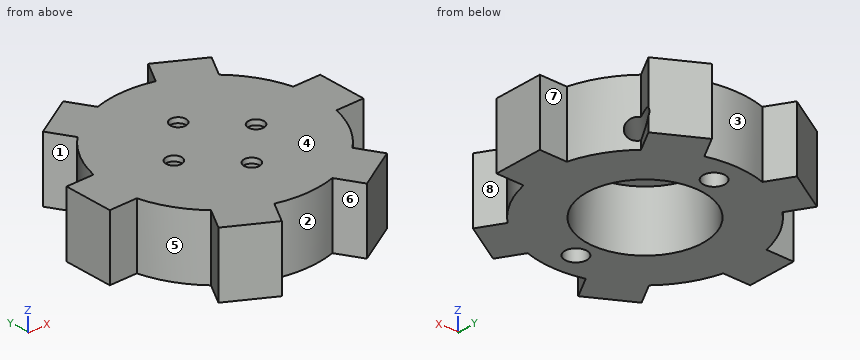
Autodesk Inventor part; units mm, degrees
ref_plane "РабПлоскость1" through (-24.7024, -23.7395, 10.5) normal (0, 0, 1) x (1, 0, 0)
ref_plane "РабПлоскость2" through (-24.7024, -23.7395, 9) normal (0, 0, -1) x (0, 1, 0)
ref_plane "YZ Plane" through (0, 0, 0) normal (1, 0, 0) x (0, 1, 0)
sketch "Эскиз1" plane through (0, 0, 0) normal (0, 0, 1) x (1, 0, 0)
  line L0 (0, 0) -> (34.5691, 5.4752) construction
  line L1 (0, 0) -> (35, 0) construction
  line L2 (0, 0) -> (34.5691, -5.4752) construction
  circle A0 centre (0, 0) radius 11.25
  circle A1 centre (0, 0) radius 15
  circle A2 centre (0, 0) radius 20
  circle A3 centre (0, 0) radius 30.0525
  circle A4 centre (0, 0) radius 32.0038
  circle A5 centre (0, 0) radius 35
  line L3 (0, 0) -> (17.5, -30.3109) construction
  circle A6 centre (0, -8) radius 1.5
  circle A7 centre (-8, 0) radius 1.5
  line L4 (0, 0) -> (-35, 0) construction
  line L5 (-29.6307, -4.693) -> (-19.4416, -4.693) construction
  line L6 (-29.6307, -4.693) -> (-19.4416, -4.693)
  line L7 (-29.6839, -4.693) -> (-29.6839, 4.693)
  line L8 (-19.4416, 4.693) -> (-34.6839, 4.693) construction
  line L9 (-19.4416, -4.693) -> (-34.6839, -4.693) construction
  line L10 (10.751, 28.0074) -> (5.6565, 19.1834) construction
  line L11 (5.6565, 19.1834) -> (13.2777, 32.3837) construction
  line L12 (-5.6565, 19.1834) -> (-13.2777, 32.3837) construction
  circle A8 centre (0, 8) radius 1.5
  line L13 (0, 0) -> (-17.5, 30.3109) construction
  line L14 (-5.6565, 19.1834) -> (-13.2777, 32.3837)
  line L15 (0, 0) -> (17.5, 30.3109) construction
  line L16 (0, 0) -> (-17.5, -30.3109) construction
  line L17 (5.6565, 19.1834) -> (13.2777, 32.3837)
  line L18 (13.3758, 26.5536) -> (16.0133, 31.1219)
  line L19 (16.3082, 24.8605) -> (18.9457, 29.4289)
  line L20 (18.9457, 29.4289) -> (17.4457, 26.8308) construction
  line L21 (29.6307, 4.693) -> (19.4416, 4.693)
  line L22 (18.8796, -23.3144) -> (13.7851, -14.4904) construction
  line L23 (13.7851, -14.4904) -> (21.4063, -27.6907) construction
  line L24 (29.6839, 4.693) -> (29.6839, 1.693)
  line L25 (29.6839, 4.693) -> (29.6839, -4.693)
  line L26 (29.6839, -4.693) -> (29.6839, -1.693) construction
  circle A9 centre (8, 0) radius 1.5
  line L27 (-18.8796, 23.3144) -> (-13.7851, 14.4904) construction
  line L28 (-13.7851, 14.4904) -> (-21.4063, 27.6907) construction
  line L29 (-18.8796, 23.3144) -> (-13.7851, 14.4904)
  line L30 (-13.7851, 14.4904) -> (-21.4063, 27.6907)
  line L31 (-18.9063, 23.3605) -> (-10.7777, 28.0536)
  line L32 (-16.3082, 24.8605) -> (-18.9457, 29.4289)
  line L33 (-13.3758, 26.5536) -> (-16.0133, 31.1219)
  line L34 (-13.7851, -14.4904) -> (-21.4063, -27.6907) construction
  line L35 (-10.751, -28.0074) -> (-5.6565, -19.1834) construction
  line L36 (-13.7851, -14.4904) -> (-21.4063, -27.6907)
  line L37 (-10.751, -28.0074) -> (-5.6565, -19.1834)
  line L38 (13.7851, 14.4904) -> (21.4063, 27.6907) construction
  line L39 (21.4063, 27.6907) -> (20.1674, 25.5449) construction
  line L40 (10.7777, 28.0536) -> (18.9063, 23.3605)
  line L41 (13.7851, 14.4904) -> (21.4063, 27.6907)
  line L42 (10.751, 28.0074) -> (5.6565, 19.1834)
  line L43 (0, 0) -> (21.2118, 27.8399) construction
  line L44 (0, 0) -> (8, 0) construction
  line L45 (0, 0) -> (0, 8) construction
  line L46 (-10.7777, -28.0536) -> (-18.9063, -23.3605)
  line L47 (-13.3758, -26.5536) -> (-16.0133, -31.1219)
  line L48 (-16.3082, -24.8605) -> (-18.9457, -29.4289)
  line L49 (-5.6565, -19.1834) -> (-13.2777, -32.3837) construction
  line L50 (5.6565, -19.1834) -> (13.2777, -32.3837) construction
  line L51 (-5.6565, -19.1834) -> (-13.2777, -32.3837)
  line L52 (18.8796, -23.3144) -> (13.7851, -14.4904)
  line L53 (5.6565, -19.1834) -> (13.2777, -32.3837)
  line L54 (16.3082, -24.8605) -> (18.9457, -29.4289)
  line L55 (13.7851, -14.4904) -> (21.4063, -27.6907)
  line L56 (13.3758, -26.5536) -> (16.0133, -31.1219)
  line L57 (18.9063, -23.3605) -> (10.7777, -28.0536)
  line L58 (27.6414, 16.1308) -> (28.831, 19.8437)
  line L59 (24.938, 20.0584) -> (28.831, 19.8437)
  line L60 (24.7499, 20.2901) -> (25.3388, 24.1443)
  line L61 (21.4607, 23.742) -> (25.3388, 24.1443)
  line L62 (17.4457, 26.8308) -> (21.2118, 27.8399)
  line L63 (21.2384, 23.9411) -> (21.2118, 27.8399)
  line L64 (-19.4416, 4.693) -> (-34.6839, 4.693)
  line L65 (-17.4453, 26.8311) -> (-21.2113, 27.8403)
  line L66 (-21.238, 23.9415) -> (-21.2113, 27.8403)
  line L67 (-21.4603, 23.7424) -> (-25.3384, 24.1447)
  line L68 (-24.7496, 20.2905) -> (-25.3384, 24.1447)
  line L69 (-24.9377, 20.0588) -> (-28.8307, 19.8442)
  line L70 (-27.6411, 16.1312) -> (-28.8307, 19.8442)
  line L71 (-27.7903, 15.8727) -> (-31.6007, 15.0465)
  line L72 (-29.8401, 11.5678) -> (-31.6007, 15.0465)
  line L73 (-29.9467, 11.289) -> (-33.5789, 9.8719)
  line L74 (-31.2916, 6.7145) -> (-33.5789, 9.8719)
  line L75 (-31.3528, 6.4224) -> (-34.716, 4.45)
  line L76 (-29.6839, -1.693) -> (-34.959, -1.693)
  line L77 (-19.4416, -4.693) -> (-34.6839, -4.693)
  line L78 (-29.6839, 1.693) -> (-34.959, 1.693)
  line L79 (-31.959, 1.693) -> (-34.716, 4.45)
  line L80 (-31.9591, -1.6925) -> (-34.716, -4.4494)
  line L81 (-31.3529, -6.4219) -> (-34.716, -4.4494)
  line L82 (-31.2917, -6.714) -> (-33.5791, -9.8714)
  line L83 (-29.9469, -11.2885) -> (-33.5791, -9.8714)
  line L84 (-29.8403, -11.5673) -> (-31.6009, -15.046)
  line L85 (-27.7906, -15.8723) -> (-31.6009, -15.046)
  line L86 (-24.938, -20.0584) -> (-28.831, -19.8437)
  line L87 (-27.6414, -16.1308) -> (-28.831, -19.8437)
  line L88 (-17.4457, -26.8308) -> (-21.2118, -27.8399)
  line L89 (-21.2384, -23.9411) -> (-21.2118, -27.8399)
  line L90 (-21.4607, -23.742) -> (-25.3388, -24.1443)
  line L91 (-24.7499, -20.2901) -> (-25.3388, -24.1443)
  line L92 (-14.5138, -28.5236) -> (-13.5047, -32.2897)
  line L93 (-10.1149, -30.3634) -> (-13.5047, -32.2897)
  line L94 (-9.8313, -30.4564) -> (-8.2407, -34.016)
  line L95 (-5.1973, -31.579) -> (-8.2407, -34.016)
  line L96 (-4.9026, -31.6261) -> (-2.7702, -34.8902)
  line L97 (-0.1495, -32.0035) -> (-2.7702, -34.8902)
  line L98 (0.149, -32.0035) -> (2.7697, -34.8902)
  line L99 (-14.5133, 28.5238) -> (-13.5042, 32.2899)
  line L100 (-10.1144, 30.3635) -> (-13.5042, 32.2899)
  line L101 (-9.8308, 30.4565) -> (-8.2401, 34.0162)
  line L102 (-5.1968, 31.5791) -> (-8.2401, 34.0162)
  line L103 (14.5138, 28.5236) -> (13.5047, 32.2897)
  line L104 (10.1149, 30.3634) -> (13.5047, 32.2897)
  line L105 (9.8313, 30.4564) -> (8.2407, 34.016)
  line L106 (5.1973, 31.579) -> (8.2407, 34.016)
  line L107 (4.9026, 31.6261) -> (2.7702, 34.8902)
  line L108 (0.1495, 32.0035) -> (2.7702, 34.8902)
  line L109 (-4.9021, 31.6262) -> (-2.7697, 34.8902)
  line L110 (-0.149, 32.0035) -> (-2.7697, 34.8902)
  line L111 (14.5133, -28.5238) -> (13.5042, -32.2899)
  line L112 (5.1968, -31.5791) -> (8.2401, -34.0162)
  line L113 (9.8308, -30.4565) -> (8.2401, -34.0162)
  line L114 (10.1144, -30.3635) -> (13.5042, -32.2899)
  line L115 (17.4453, -26.8311) -> (21.2113, -27.8403)
  line L116 (21.238, -23.9415) -> (21.2113, -27.8403)
  line L117 (4.9021, -31.6262) -> (2.7697, -34.8902)
  line L118 (19.4416, -4.693) -> (34.6839, -4.693)
  line L119 (29.6839, -1.693) -> (34.959, -1.693)
  line L120 (21.4603, -23.7424) -> (25.3384, -24.1447)
  line L121 (24.7496, -20.2905) -> (25.3384, -24.1447)
  line L122 (24.9377, -20.0588) -> (28.8307, -19.8442)
  line L123 (27.6411, -16.1312) -> (28.8307, -19.8442)
  line L124 (27.7903, -15.8727) -> (31.6007, -15.0465)
  line L125 (29.9467, -11.289) -> (33.5789, -9.8719)
  line L126 (31.2916, -6.7145) -> (33.5789, -9.8719)
  line L127 (31.3528, -6.4224) -> (34.716, -4.45)
  line L128 (31.959, -1.693) -> (34.716, -4.45)
  line L129 (29.8401, -11.5678) -> (31.6007, -15.0465)
  line L130 (34.5691, 5.4752) -> (29.6307, 4.693) construction
  line L131 (19.4416, 4.693) -> (34.6839, 4.693)
  line L132 (34.6839, 4.693) -> (29.6839, 4.693) construction
  line L133 (29.6839, 1.693) -> (34.959, 1.693)
  line L134 (29.8403, 11.5673) -> (31.6009, 15.046)
  line L135 (31.2917, 6.714) -> (33.5791, 9.8714)
  line L136 (31.9591, 1.6925) -> (34.716, 4.4494)
  line L137 (31.3529, 6.4219) -> (34.716, 4.4494)
  line L138 (29.9469, 11.2885) -> (33.5791, 9.8714)
  line L139 (27.7906, 15.8723) -> (31.6009, 15.046)
  circle A10 centre (0, 0) radius 36.5
  line L140 (0, 0) -> (-24.7487, 24.7487) construction
  line L141 (0, 0) -> (35, 0) construction
  line L142 (0, 0) -> (-24.6962, 0) construction
  line L143 (-24.6962, -4.693) -> (-24.6962, 4.693)
  line L144 (-8.2838, -23.734) -> (-16.4124, -19.041)
  line L145 (16.4124, -19.041) -> (8.2838, -23.734)
  line L146 (24.6962, 4.693) -> (24.6962, -4.693)
  line L147 (8.2838, 23.734) -> (16.4124, 19.041)
  line L148 (-16.4124, 19.041) -> (-8.2838, 23.734)
  line L149 (0, 0) -> (21.2503, 21.2503) construction
  line L150 (0, 0) -> (30.0525, 0) construction
  line L151 (14.1421, 14.1421) -> (23.5912, 4.693)
  line L152 (23.5912, 4.693) -> (-6.168, 34.4522)
  circle A11 centre (0, 15) radius 2.1
  circle A12 centre (0, -15) radius 2.1
  point P0 (0, 0)
  point P1 (18.9062, 23.3604)
  point P2 (18.9055, 23.3609)
  point P3 (10.7784, 28.0531)
  point P4 (-10.7784, 28.0531)
  point P5 (-18.9055, 23.3609)
  point P6 (-18.9062, 23.3604)
  point P7 (-29.6838, 4.693)
  point P8 (-29.6839, 4.6922)
  point P9 (-29.6839, -4.6922)
  point P10 (-18.9055, -23.3609)
  point P11 (-10.7784, -28.0531)
  point P12 (-10.7776, -28.0534)
  point P13 (10.7776, -28.0534)
  point P14 (10.7784, -28.0531)
  point P15 (18.9055, -23.3609)
  point P16 (29.6839, -4.6922)
  point P17 (29.6839, 4.6922)
  point P18 (29.6838, 4.693)
  point P19 (-29.6838, -4.693)
  point P20 (-18.9062, -23.3604)
  point P21 (18.9062, -23.3604)
  point P22 (29.6838, -4.693)
  point P23 (10.7776, 28.0534)
  point P24 (-10.7776, 28.0534)
  point P25 (-24.6962, 4.693)
  point P26 (24.6962, -4.693)
  dimension "d10" = 70
  dimension "d21" = 60.105
  dimension "d31" = 30
  dimension "d11" = 40
  dimension "d12" = 9
  dimension "d13" = 5
  dimension "d14" = 360
  dimension "d15" = 360
  dimension "d16" = 5
  dimension "d17" = 90
  dimension "d18" = 3
  dimension "d19" = 3
  dimension "d20" = 360
  dimension "d22" = 3
  dimension "d23" = 45
  dimension "d24" = 45.392
  dimension "d25" = 360
  dimension "d26" = 22.5
  dimension "d27" = 8
  dimension "d28" = 3
  dimension "d29" = 8
  dimension "d30" = 3
  dimension "d32" = 73
  dimension "d45" = 135
  dimension "d48" = 360
  dimension "d54" = 45
  dimension "d63" = 4.2
extrude "Выдавливание1" add sketch "Эскиз1" along normal blind 11.5 contours A1 A12 A11 | A11 A1 | A1 A11 | A12 A1 | A1 A12 | A2
extrude "Выдавливание4" add sketch "Эскиз1" along normal blind 1 from surface at 11.5 contours A0 | A1 A12 A11 | A11 A1 | A1 A11 | A12 A1 | A1 A12 | A2
ref_plane "РабПлоскость1" through (-24.7024, -23.7395, 10.5) normal (0, 0, 1) x (1, 0, 0)
ref_plane "РабПлоскость2" through (-24.7024, -23.7395, 9) normal (0, 0, -1) x (0, 1, 0)
extrude "Выдавливание7" add sketch "Эскиз1" along normal blind 12.5 contours A2 L21 L146 L118 | L52 L145 L53 A2 | A2 L17 L152 L41 | L152 L17 L147 L41 | L37 L144 L36 A2 | A2 L29 L148 L14 | L6 L143 L64 A2
ref_plane "РабПлоскость3" through (23.5912, 4.693, 0) normal (0.7071068, 0.7071068, 0) x (-0.7071068, 0.7071068, 0)
sketch "Эскиз2" plane through (23.5912, 4.693, 0) normal (0.7071068, 0.7071068, 0) x (-0.7071068, 0.7071068, 0)
  line L0 (13.363, 0) -> (13.363, 3.5)
  line L1 (13.8618, 0) -> (13.8618, 12.5)
  line L2 (13.363, 0) -> (16.863, 0) construction
  circle A0 centre (13.363, 3.5) radius 2
  dimension "d56" = 3.5
  dimension "d57" = 90
  dimension "d58" = 4
extrude "Выдавливание8" cut sketch "Эскиз2" along normal blind 5.1 and the other way blind 9
sketch "Эскиз3" plane through (0, 0, 0) normal (0, 0, -1) x (-1, 0, 0)
  point P0 (0, 0)
extrude "Выдавливание9" cut sketch "Эскиз1" along normal blind 6 contours A0 | A11 A1 | A1 A11 | A12 A1 | A1 A12 | A6 | A7 | A8 | A9
properties part number "inside_part_wheel"
Read the model definition and answer for the solid it produces. Units are mm, in the model's axes. Face numbers are marked on the shaded views. A direction names the side the tool comes from. Give positions to 0.01 mm unless a question says otherwise; leave off trailing zeros. Write each loop counter-clockwise with the first axis right and the second up, starting at its lowest first coordinate (ties: lowest second). Pieces come first, ordered by that corner, then holes. Notation, with made-up numbers: (-27.5, 89) - (-4.5, 89) arc R23 cw to (-4.5, 123) - close; hole circle Ø4 at (-8.5, 87). An arc over 180 degrees is marked (long way). Answer in a Markdown table with one row per item. Add a question column.
Item 1: Section B-B, the plane x = 21.5 is taken. Write down the section's boundary in (y, z), and give its area (3 significant figures).
Item 2: Find the intervals of material crossed by L1, parallel to Y at x = -1.5, z = 0.5; L2, parallel to Y at x = -15.5, z = 4; L3, parallel to X at y = -15.5, z = 2.75, in increasing order.
Item 3: Section C-C, the plane y = -18 is taken. Write down the section's boundary in (x, z).
Item 4: Determine the mould class of the marked faces 1, 2, 3 and 4 for opening direction X: pulls with the +X half, pulls with the -X half, needs draft (parallel to the pull), parting line crosses it, or undercut.
Item 5: Flat-ended cylindrical pins translate along their axes: P1, Ø11, axis at x = -5, y = -1.5, coming from the -Z side; P2, Ø6, axis at x = -23, z = 8.5, coming from the -Y side; P3, Ø3, axis at x = -3, z = 10.5, coming from the -Y side. Find the tip coordinate at first contact, or state that the pin passes through.
Item 6: A tool of negligible diameter and unlimited length cuts with its end or side. For the marked faces 5, 6, 7 and 8, from which of +Z, -Z, +X, -X, +Y, -Y can it reach the whole face along a straight path? Write none if from no direction.
Item 7: Section A-A, the plane z = 9.25 is taken. Write down the section's boundary in (x, y), and give its area (3 significant figures).
Recorded:
| question | item | result |
|---|---|---|
| 1 | outline | (-4.69, 0) - (4.69, 0) - (4.69, 12.5) - (-4.69, 12.5) - close |
| 1 | area | 117 mm2 |
| 2 | L1 | y = -19.94 to -16.47, -13.53 to -11.15, 11.15 to 13.53, 16.47 to 19.94 |
| 2 | L2 | y = -19.57 to -17.46, -12.64 to 12.64, 17.46 to 19.57 |
| 2 | L3 | x = -14.37 to -2.04, 2.04 to 14.37 |
| 3 | outline | (-15.81, 0) - (15.81, 0) - (15.81, 12.5) - (-15.81, 12.5) - close |
| 4 | face 1 | pulls with the -X half |
| 4 | face 2 | undercut |
| 4 | face 3 | undercut |
| 4 | face 4 | needs draft |
| 5 | P1 | stops at z = 11.5 |
| 5 | P2 | stops at y = -4.69 |
| 5 | P3 | stops at y = -19.94 |
| 6 | face 5 | +Z, -Z, -X |
| 6 | face 6 | +Z, -Z, -Y |
| 6 | face 7 | +Z, -Z, +X, +Y |
| 6 | face 8 | +Z, -Z, +X |
| 7 | outline | (-24.7, -4.69) - (-19.44, -4.69) arc R20 ccw to (-13.79, -14.49) - (-16.41, -19.04) - (-8.28, -23.73) - (-5.66, -19.18) arc R20 ccw to (5.66, -19.18) - (8.28, -23.73) - (16.41, -19.04) - (13.79, -14.49) arc R20 ccw to (19.44, -4.69) - (24.7, -4.69) - (24.7, 4.69) - (19.44, 4.69) arc R20 ccw to (13.79, 14.49) - (16.41, 19.04) - (8.28, 23.73) - (5.66, 19.18) arc R20 ccw to (-5.66, 19.18) - (-8.28, 23.73) - (-16.41, 19.04) - (-13.79, 14.49) arc R20 ccw to (-19.44, 4.69) - (-24.7, 4.69) - close; hole circle Ø22.5 at (0, 0) |
| 7 | area | 1,130 mm2 |
